Part model, mm, in its own coordinate system. A direction names the side the tool comes from. Coordinates: 2 decimals unless noted, no trailing zeros. Loops run counter-clockwise (first coordinate to the right, second up) from the corner with the lowest first, then second, coordinate; pieces in that order, holes last. Notation, with made-up numbers: M 69,21 L 76,21 A20 cw 76,43 Z; hole C 27.25,25 d3. An arc over 180 degrees is marked long. Use a Markdown table: item, result. Add a question column.
1) Wall check: probe 1 along Y at (x, z) = (0, -1.5) (1 decimal); probe 2 along Y at (x, z) = (19.5, -19.25); probe 3 along X at (y, z) = (6.5, -9.25). Give the ranges that are in metal, low to high. Write a range as from..to.
2) Band-saw the part on C-C (z = 1.25). List the corners of the cut face in (x, y), plus the area to 3 significant figures.
3) Band-saw the part on B-B (y = 37.5). List the corners of the cut face in (x, z), plus the area to 3 significant figures.
4) Tool access for faces 1 (the flat face through (-1, 38, 3)), 2 (the cylindrical face through (34.242, 2.433, -10.846)): list every direction of +Z, -Z, +X, -X, +Y, -Y with a clear straight run to the whole face (end or side of a thin tool).
5) Band-saw the part on A-A (x = 0). List the corners of the cut face in (y, z) (1 decimal).
6) Pin check, flat tips, straight feed: pin 1 Ø1 at (x, y) = (-1.5, 34) entering from -Z; pin 2 Ø6 at (x, y) = (0, 64.02) entering from -Z; pin 3 Ø8 at (x, z) = (-26, -8) entering from -Y; pin 4 Ø3 at (y, z) = (3.5, -12.5) entering from -X. Stop position of each tip, or through.
7) Band-saw the part on D-D (z = -11.5). State how many separate pieces and enclosed holes the cut face has, plus the area to 3 significant figures.
8) Pull direction Y, two halves, no side cores. Call faces 3 (the flat face through (-50, 37, -11)), 4 (the cylindrical face through (-41.445, 78.479, -11.196)), 5 (the flat face through (26, 64, 0)), 6 (the cylindrical face through (40.979, -3.945, -10.804)): released by +Y, released by -Y, zero draft, split by the parting line, or undercut.
from build123d import *

# Parameters (mm, degrees)
SKETCH1_W           = 100
SKETCH1_H           = 100
SKETCH1_R           = 4.025
SKETCH1_R_2         = 8.1
BOSS_EXTRUDE1_DEPTH = 25
SKETCH2_W           = 100
SKETCH2_H           = 100
SKETCH2_R           = 5
BOSS_EXTRUDE2_DEPTH = 3
FILLET1_R           = 30
FILLET2_R           = 3
SKETCH3_R           = 7.5
CUT_EXTRUDE1_DEPTH  = 25
FILLET3_R           = 3


with BuildPart() as part:
    # Sketch1 → Boss-Extrude1 (new body)
    with BuildSketch(Plane.XY):
        with Locations((0, 37.5)):
            Rectangle(SKETCH1_W, SKETCH1_H)
        Circle(SKETCH1_R, mode=Mode.SUBTRACT)
        with Locations((26.516504294, 64.016504294)):
            Circle(SKETCH1_R, mode=Mode.SUBTRACT)
        with Locations((-26.516504294, 64.016504294)):
            Circle(SKETCH1_R, mode=Mode.SUBTRACT)
        with Locations((0, 64.016504294)):
            Circle(SKETCH1_R_2, mode=Mode.SUBTRACT)
        with Locations((-26.516504294, 0)):
            Circle(SKETCH1_R_2, mode=Mode.SUBTRACT)
        with Locations((26.516504294, 0)):
            Circle(SKETCH1_R_2, mode=Mode.SUBTRACT)
    extrude(amount=-BOSS_EXTRUDE1_DEPTH)

    # Sketch2 → Boss-Extrude2 (add)
    with BuildSketch(Plane.XY):
        with Locations((0, 37.5)):
            Rectangle(SKETCH2_W, SKETCH2_H)
        with Locations((0, 64.016504294)):
            Circle(SKETCH2_R, mode=Mode.SUBTRACT)
        with Locations((26.516504294, 0)):
            Circle(SKETCH2_R, mode=Mode.SUBTRACT)
        with Locations((-26.516504294, 0)):
            Circle(SKETCH2_R, mode=Mode.SUBTRACT)
    extrude(amount=BOSS_EXTRUDE2_DEPTH)

    # Fillet1
    fillet1_edges = [part.edges().sort_by_distance(p)[0] for p in [
        (-50, 87.5, -11),
        (50, 87.5, -11),
        (50, -12.5, -11),
        (-50, -12.5, -11),
    ]]
    fillet(fillet1_edges, radius=FILLET1_R)

    # Fillet2
    fillet2_edges = [part.edges().sort_by_distance(p)[0] for p in [
        (-8.1, 64.016504294, -25),
        (-34.616504294, 0, -25),
        (18.416504295, 0, -25),
    ]]
    fillet(fillet2_edges, radius=FILLET2_R)

    # Sketch3 → Cut-Extrude1 (cut)
    with BuildSketch(Plane(origin=(0, 0, -25), x_dir=(-1, 0, 0), z_dir=(0, 0, -1))):
        with Locations((0, 37.5)):
            Circle(SKETCH3_R)
    extrude(amount=-CUT_EXTRUDE1_DEPTH, mode=Mode.SUBTRACT)

    # Fillet3
    fillet3_edges = [part.edges().sort_by_distance(p)[0] for p in [
        (7.5, 37.5, -25),
    ]]
    fillet(fillet3_edges, radius=FILLET3_R)


solid = part.part
Entries:
| question | item | result |
|---|---|---|
| 1 | probe 1 | -12.5..-4, 4..30, 45..55.9, 72.1..87.5 |
| 1 | probe 2 | -12.5..-4.05, 4.05..87.5 |
| 1 | probe 3 | -47.91..-31.35, -21.68..21.68, 31.35..47.91 |
| 2 | outline | M -50,17.5 A30 ccw -20,-12.5 L 20,-12.5 A30 ccw 50,17.5 L 50,57.5 A30 ccw 20,87.5 L -20,87.5 A30 ccw -50,57.5 Z; hole C -26.52,0 d10; hole C 0,64.02 d10; hole C 26.52,0 d10 |
| 2 | area | 8,990 mm2 |
| 3 | outline | M -50,-25 L -10.5,-25 A3 ccw -7.5,-22 L -7.5,0 L 7.5,0 L 7.5,-22 A3 ccw 10.5,-25 L 50,-25 L 50,3 L -50,3 Z |
| 3 | area | 2,420 mm2 |
| 4 | face 1 | +Z, +X, -X, +Y, -Y |
| 4 | face 2 | -Z |
| 5 | outline | M -12.5,-25 L -4,-25 L -4,0 L 4,0 L 4,-25 L 27,-25 A3 ccw 30,-22 L 30,0 L 45,0 L 45,-22 A3 ccw 48,-25 L 52.9,-25 A3 ccw 55.9,-22 L 55.9,0 L 59,0 L 59,3 L -12.5,3 Z; M 69,0 L 72.1,0 L 72.1,-22 A3 ccw 75.1,-25 L 87.5,-25 L 87.5,3 L 69,3 Z |
| 6 | pin 1 | z = 0 |
| 6 | pin 2 | through |
| 6 | pin 3 | y = -12.43 |
| 6 | pin 4 | x = -47.27 |
| 7 | separate pieces | 1 |
| 7 | enclosed holes | 7 |
| 7 | area | 8,280 mm2 |
| 8 | face 3 | zero draft |
| 8 | face 4 | released by +Y |
| 8 | face 5 | undercut |
| 8 | face 6 | released by -Y |
